Check sheet for the drawn part. Datum: minimum x, y, z corner. Units: mm. Round coordinates to 2 decimals unless told otherwise and drop trailing zeros. Write each loop counter-clockwise with the first axis right and the second up, starting at its lowest first coordinate (ties: lowest second). Pieces come first, ordered by that corner, then holes. Notation, with made-up numbers: (53, -28) - (81, -28) arc R21 ccw to (81, 3) - close; hole circle Ø4 at (57.5, -14). An arc over 180 degrees is marked (long way). Write each question's results on one line, items separated by ' | '.
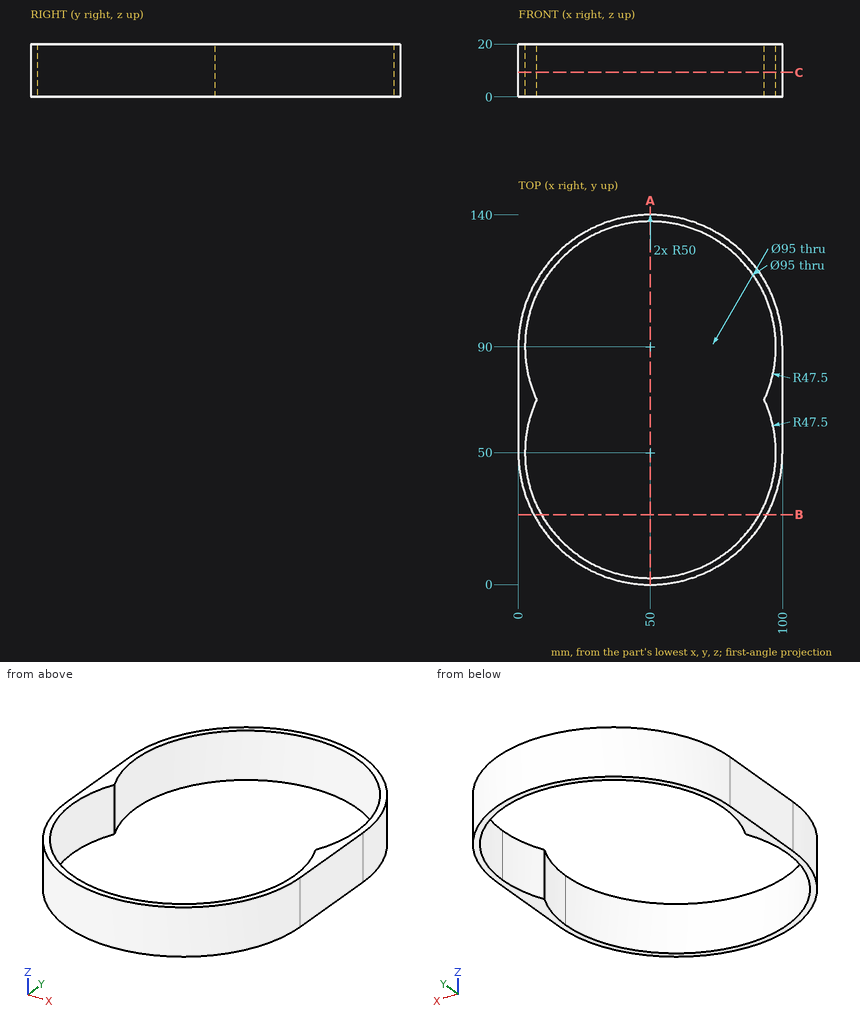
(1) Section check B-B (y = 26.5). Record the cut outline in (x, z), plus the area to 3 significant figures.
Answer:
outline: (5.87, 0) - (8.72, 0) - (8.72, 20) - (5.87, 20) - close; (91.28, 0) - (94.13, 0) - (94.13, 20) - (91.28, 20) - close | area: 114 mm2
(2) Section check C-C (z = 9.25). Record the cut outline in (x, y), plus the area to 3 significant figures.
Answer:
outline: (0, 50) arc R50 ccw to (100, 50) - (100, 90) arc R50 ccw to (0, 90) - close; hole (6.92, 70) arc R47.5 ccw (long way) to (93.08, 70) arc R47.5 ccw (long way) to start | area: 1,080 mm2
(3) Section check A-A (x = 50). Record the cut outline in (y, z).
Answer:
outline: (0, 0) - (2.5, 0) - (2.5, 20) - (0, 20) - close; (137.5, 0) - (140, 0) - (140, 20) - (137.5, 20) - close
(4) Go/stop test with flat-tipped pins: pin 1 Ø4 at (x, z) = (60.5, 12.5) entering from -Y; pin 2 Ø5 at (x, z) = (52, 8) entering from +Y. Record where each tip stops, or that it passes through.
Answer:
pin 1: y = 0.73 | pin 2: y = 140
(5) Thickness scan on L1, parallel to Y at x = 50, z = 7.5; L2, parallel to X at y = 50, z = 12.5; L3, parallel to Y at x = 63.5, z = 1.75. Record the ranges inside material, lowest first.
Answer:
L1: 0 to 2.5, 137.5 to 140 | L2: 0 to 2.5, 97.5 to 100 | L3: 1.86 to 4.46, 135.54 to 138.14
